```python
from build123d import *

# Parameters (mm, degrees)
IZIM1_W                     = 60
IZIM1_H                     = 11
Y_KSEKLIK_EKSTR_ZYON1_DEPTH = 210
KES_EKSTR_ZYON1_DEPTH       = 213.996779223
KES_EKSTR_ZYON1_DEPTH_BACK  = 213.996779223
IZIM2_R                     = 14.14
IZIM2_R_2                   = 2.3
IZIM3_R                     = 1.4
KES_EKSTR_ZYON2_DEPTH       = 21
KES_EKSTR_ZYON3_START       = -21
IZIM4_R                     = 1.4
KES_EKSTR_ZYON3_DEPTH       = 21


with BuildPart() as part:
    # Çizim1 → Yükseklik-Ekstrüzyon1 (new body)
    with BuildSketch(Plane.XY):
        with Locations((3.861895391, 4.551835536)):
            Rectangle(IZIM1_W, IZIM1_H)
    extrude(amount=Y_KSEKLIK_EKSTR_ZYON1_DEPTH)

    # Çizim2 → Kes-Ekstrüzyon1 (cut, two sides: drawn at the far end of the back side and taken through both)
    with BuildSketch(Plane(origin=(0, 10.051835536, 0), x_dir=(1, 0, 0), z_dir=(0, 1, 0)).offset(-KES_EKSTR_ZYON1_DEPTH_BACK)):
        with Locations(Location((3.861895391, -105.86, 0), (0, 0, 270))):
            Circle(IZIM2_R)
        with Locations(Location((-10.278104609, -91.72, 0), (0, 0, 270))):
            Circle(IZIM2_R_2)
        with Locations(Location((18.001895391, -91.72, 0), (0, 0, 270))):
            Circle(IZIM2_R_2)
        with Locations(Location((18.001895391, -120, 0), (0, 0, 270))):
            Circle(IZIM2_R_2)
        with Locations(Location((-10.278104609, -120, 0), (0, 0, 270))):
            Circle(IZIM2_R_2)
    extrude(amount=KES_EKSTR_ZYON1_DEPTH + KES_EKSTR_ZYON1_DEPTH_BACK, mode=Mode.SUBTRACT)

    # Çizim3 → Kes-Ekstrüzyon2 (cut)
    with BuildSketch(Plane(origin=(0, 0, 0), x_dir=(-1, 0, 0), z_dir=(0, 0, -1))):
        with Locations((21.138104609, 4.551835536)):
            Circle(IZIM3_R)
        with Locations((-28.861895391, 4.551835536)):
            Circle(IZIM3_R)
    extrude(amount=-KES_EKSTR_ZYON2_DEPTH, mode=Mode.SUBTRACT)

    # Çizim4 → Kes-Ekstrüzyon3 (cut)
    with BuildSketch(Plane.XY.offset(210).offset(KES_EKSTR_ZYON3_START)):
        with Locations(Location((-21.138104609, 4.551835536, 0), (0, 0, 180))):
            Circle(IZIM4_R)
        with Locations(Location((28.861895391, 4.551835536, 0), (0, 0, 180))):
            Circle(IZIM4_R)
    extrude(amount=KES_EKSTR_ZYON3_DEPTH, mode=Mode.SUBTRACT)


solid = part.part
```
Check sheet for the modelled part. Datum: model origin and axes. Units: mm. Coordinates: 2 decimals unless noted, no trailing zeros. Loops run counter-clockwise (first coordinate to the right, second up) from the corner with the lowest first, then second, coordinate; pieces in that order, holes last.
1) Material ranges on probe 1 along Z at (x, y) = (18.5, 5.25); probe 2 along Z at (x, y) = (-11.5, 1); probe 3 along X at (y, z) = (5.25, 101), recorded low to high.
2) Release check for a two-part mould opening along Z. For faces 1 (the face through (-11.159, 4.475, 93.845)), 2 (the face through (3, 5, 210)), 3 (the face through (-26.138, 4, 104)) record: released by +Z, released by -Z, zero draft, split by the parting line, or undercut.
3) Gauge pin test, flat ends, axial feed: pin 1 (1.7 mm diameter, centred on x = -21.14, y = 4.55, fed in from -Z); pin 2 (0.8 mm diameter, centred on x = 28.5, y = 5, fed in from +Z). Record the tip position at first contact, or that the pin passes through.
4) Sectioned sample at A-A (z = 105.86). Record the boundary of the cut face in (x, y), and give its area (3 significant figures).
5) Sectioned sample at B-B (x = -0.5). Record the boundary of the cut face in (y, z), and give its area (3 significant figures).
Check sheet entries:
1. probe 1: z = 0 to 89.47, 93.97 to 117.75, 122.25 to 210
1. probe 2: z = 0 to 89.77, 93.67 to 118.05, 121.95 to 210
1. probe 3: x = -26.14 to -9.42, 17.14 to 33.86
2. face 1: undercut
2. face 2: released by +Z
2. face 3: zero draft
3. pin 1: stops at z = 21
3. pin 2: stops at z = 189
4. outline: (-26.14, -0.95) - (-10.28, -0.95) - (-10.28, 10.05) - (-26.14, 10.05) - close; (18, -0.95) - (33.86, -0.95) - (33.86, 10.05) - (18, 10.05) - close
4. area: 349 mm2
5. outline: (-0.95, 0) - (10.05, 0) - (10.05, 92.41) - (-0.95, 92.41) - close; (-0.95, 119.31) - (10.05, 119.31) - (10.05, 210) - (-0.95, 210) - close
5. area: 2,010 mm2
